Verification items for the finished model (mm, model axes). A direction names the side the tool comes from. Coordinates: 2 decimals unless noted, no trailing zeros. Order: outer loops, then holes, each group sorted by start corner. A loop starts at its lowest first (then second) coordinate and runs counter-clockwise, first axis right, second up. Notation, with made-up numbers: (73, -32.5) - (95, -32.5) arc R19 cw to (95, -8.5) - close; hole circle Ø8 at (-6, -35.5). An arc over 180 degrees is marked (long way). Answer as CSV lines item,"result". Start each with the question number.
1. Section check C-C (y = 14.5). Record the cut outline in (x, z), and give its area (3 significant figures).
2. Section check B-B (y = 8). Record the cut outline in (x, z).
3. Material ranges on L1, parallel to Y at x = 26.5, z = 16; L2, parallel to X at y = 5, z = 15; L3, parallel to Z at x = -24, y = 12.75, recorded low to high. Write a range as [from, to].
4. Go/stop test with flat-tipped pins: pin 1 (4 mm diameter, centred on y = 12.5, z = -14, fed in from +X); pin 2 (3 mm diameter, centred on y = 8, z = 11, fed in from +X); pin 3 (2 mm diameter, centred on y = 5, z = -6.5, fed in from -X); pin 4 (6 mm diameter, centred on x = -26.5, y = 8, fed in from +Z). Record where each tip stops, or that it passes through.
5. Set-up check for faces 4 (the flat face through (0, 16, 8)), 5 (the flat face through (26, 4, 11.5)), 6 (the flat face through (-22.6, 7.9, 11.5)): record each of +Z, -Z, +X, -X, +Y, -Y from which the full face is reachable in a straight line by a thin tool's end or side.
6. Section check D-D (z = 14). Record the cut outline in (x, y), and give its area (3 significant figures).
7. Section check A-A (x = 26.5). Record the cut outline in (y, z), and give its area (3 significant figures).
8. Mould release check, pull along X, two halves, no side actions. Record for faces 1 (the cylindrical face through (30.094, 8.158, 14.458)), 2 (the flat face through (0, 8, 17.5)), 3 (the flat face through (-17.963, 7.888, 4.946)): pulls with the +X half, pulls with the -X half, needs draft (parallel to the pull), parting line crosses it, or undercut.
from build123d import *

# Parameters (mm, degrees)
SKETCH_1_R          = 17.5
EXTRUDE_1_DEPTH     = 16
SKETCH_2_R          = 5
CUT_EXTRUDE_1_DEPTH = 16
SKETCH_3_R          = 3.597024537
CUT_EXTRUDE_2_DEPTH = 16


with BuildPart() as part:
    # 草图1 → 凸台-拉伸1 (new body)
    with BuildSketch(Plane(origin=(0, 0, 0), x_dir=(1, 0, 0), z_dir=(0, 1, 0))):
        Circle(SKETCH_1_R)
        with BuildLine():
            Line((-33.5, -11.5), (-33.5, -17.5))
            Line((-33.5, -17.5), (-7.2e-08, -17.5))
            ThreePointArc((-7.2e-08, -17.5), (-12.869300221, -11.85879892), (-17.441650698, 1.427872863))
            Line((-17.441650698, 1.427872863), (-18.5, -11.5))
            Line((-18.5, -11.5), (-33.5, -11.5))
        make_face()
        with BuildLine():
            ThreePointArc((17.5, 0), (12.374368645, -12.374368696), (-7.2e-08, -17.5))
            Line((-7.2e-08, -17.5), (33.5, -17.5))
            Line((33.5, -17.5), (33.5, -11.5))
            Line((33.5, -11.5), (18.5, -11.5))
            Line((18.5, -11.5), (17.441650698, 1.427872863))
            ThreePointArc((17.441650698, 1.427872863), (17.48540659, 0.714532286), (17.5, 0))
        make_face()
    extrude(amount=EXTRUDE_1_DEPTH)

    # 草图2 → 切除-拉伸1 (cut)
    with BuildSketch(Plane(origin=(0, 16, 0), x_dir=(1, 0, 0), z_dir=(0, 1, 0))):
        with Locations(Location((0, 0, 0), (0, 0, 270))):
            Circle(SKETCH_2_R)
    extrude(amount=-CUT_EXTRUDE_1_DEPTH, mode=Mode.SUBTRACT)

    # 草图3 → 切除-拉伸2 (cut)
    with BuildSketch(Plane(origin=(0, 0, 11.5), x_dir=(-1, 0, 0), z_dir=(0, 0, -1))):
        with Locations((-26.5, 8)):
            Circle(SKETCH_3_R)
        with Locations((26.5, 8)):
            Circle(SKETCH_3_R)
    extrude(amount=-CUT_EXTRUDE_2_DEPTH, mode=Mode.SUBTRACT)


solid = part.part
Evaluation:
1,outline,"(-33.5, 11.5) - (-18.5, 11.5) - (-17.44, -1.43) arc R17.5 ccw to (17.44, -1.43) - (18.5, 11.5) - (33.5, 11.5) - (33.5, 17.5) - (-33.5, 17.5) - close; hole circle Ø10 at (0, 0)"
1,area,"1,220 mm²"
2,outline,"(-33.5, 11.5) - (-30.1, 11.5) - (-30.1, 17.5) - (-33.5, 17.5) - close; (-22.9, 11.5) - (-18.5, 11.5) - (-17.44, -1.43) arc R17.5 ccw to (17.44, -1.43) - (18.5, 11.5) - (22.9, 11.5) - (22.9, 17.5) - (-22.9, 17.5) - close; (30.1, 11.5) - (33.5, 11.5) - (33.5, 17.5) - (30.1, 17.5) - close; hole circle Ø10 at (0, 0)"
3,L1,"y = [0, 4.4], [11.6, 16]"
3,L2,"x = [-33.5, -28.48], [-24.52, 24.52], [28.48, 33.5]"
3,L3,"z = [11.5, 17.5]"
4,pin 1,"stops at x = 12.74"
4,pin 2,"stops at x = 33.5"
4,pin 3,"stops at x = -16.61"
4,pin 4,"passes through"
5,face 4,"+Z, -Z, +X, -X, +Y"
5,face 5,"-Z, +X, +Y, -Y"
5,face 6,"-Z, -X, +Y, -Y"
6,outline,"(-33.5, 0) - (33.5, 0) - (33.5, 16) - (-33.5, 16) - close; hole circle Ø7.19 at (-26.5, 8); hole circle Ø7.19 at (26.5, 8)"
6,area,"991 mm²"
7,outline,"(0, 11.5) - (4.4, 11.5) - (4.4, 17.5) - (0, 17.5) - close; (11.6, 11.5) - (16, 11.5) - (16, 17.5) - (11.6, 17.5) - close"
7,area,"52.8 mm²"
8,face 1,"undercut"
8,face 2,"needs draft"
8,face 3,"pulls with the -X half"
